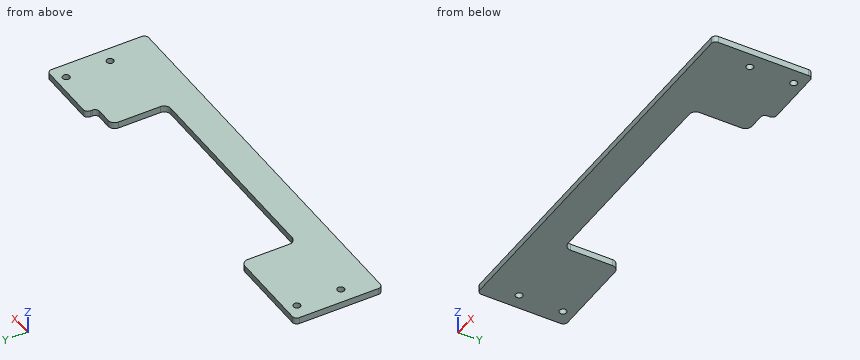
```python
from build123d import *

# Parameters (mm, degrees)
EXTRUDE_1_DEPTH     = 3
FILLET_1_R          = 2
SKETCH_2_R          = 1.6
CUT_EXTRUDE_1_DEPTH = 14
SKETCH_3_W          = 100
SKETCH_3_H          = 25
CUT_EXTRUDE_2_DEPTH = 14
FILLET_2_R          = 3


with BuildPart() as part:
    # 草图1 → 凸台-拉伸1 (new body)
    with BuildSketch(Plane.XY):
        Polygon((0, 0), (183.3, 0), (183.3, 40), (183.3, 45), (153.3, 45), (153.3, 40), (0, 40), align=None)
    extrude(amount=EXTRUDE_1_DEPTH)

    # 圆角1
    fillet_1_edges = [part.edges().sort_by_distance(p)[0] for p in [
        (0, 40, 1.5),
        (153.3, 40, 1.5),
        (153.3, 45, 1.5),
        (183.3, 45, 1.5),
        (183.3, 0, 1.5),
        (0, 0, 1.5),
    ]]
    fillet(fillet_1_edges, radius=FILLET_1_R)

    # 草图2 → 切除-拉伸1 (cut)
    with BuildSketch(Plane(origin=(0, 0, 0), x_dir=(-1, 0, 0), z_dir=(0, 0, -1))):
        with Locations((-176.3, 40.44)):
            Circle(SKETCH_2_R)
        with Locations((-176.3, 20.44)):
            Circle(SKETCH_2_R)
        with Locations((-7, 35)):
            Circle(SKETCH_2_R)
        with Locations((-7, 15)):
            Circle(SKETCH_2_R)
    extrude(amount=-CUT_EXTRUDE_1_DEPTH, mode=Mode.SUBTRACT)

    # 草图3 → 切除-拉伸2 (cut)
    with BuildSketch(Plane(origin=(0, 0, 0), x_dir=(-1, 0, 0), z_dir=(0, 0, -1))):
        with Locations((-91.65, 27.5)):
            Rectangle(SKETCH_3_W, SKETCH_3_H)
    extrude(amount=-CUT_EXTRUDE_2_DEPTH, mode=Mode.SUBTRACT)

    # 圆角2
    fillet_2_edges = [part.edges().sort_by_distance(p)[0] for p in [
        (141.65, 15, 1.5),
        (141.65, 40, 1.5),
        (41.65, 40, 1.5),
        (41.65, 15, 1.5),
    ]]
    fillet(fillet_2_edges, radius=FILLET_2_R)


solid = part.part
```
Design review of the part built by this model. Coordinates are the model's own, in mm. Coordinates: 2 decimals unless noted, no trailing zeros. Order: outer loops, then holes, each group sorted by start corner. A loop starts at its lowest first (then second) coordinate and runs counter-clockwise, first axis right, second up. Notation, with made-up numbers: M 70,-32.5 L 126,-32.5 A13 ccw 126,-26.5 Z; hole C 26.5,43.5 d3. An arc over 180 degrees is marked long. Answer as a JSON object with one key per item and string values. Group by question number.
1) Add section B-B, the plane y = 31. Write out the cut boundary in (x, z).
2) For pin 1 (1 mm diameter, centred on x = 117, z = 2.5, fed in from +Y); pin 2 (0.9 mm diameter, centred on x = 149, z = 1.5, fed in from +Y), all flat-tipped, find the tip position at first contact; note any pin that passes through.
3) Wall thickness on L1, parallel to Y at x = 176.3, z = 1.4; L2, parallel to X at y = 34.5, z = 1.7; L3, parallel to X at y = 34, z = 2.15: over which ranges is each line inside the solid? List them lowest first.
4) Add section A-A, the plane x = 7. Write out the cut boundary in (y, z).
5) Add section C-C, the plane z = 1.85. Write out the cut boundary in (x, y).
6) Add section D-D, the plane x = 176.3. Write out the cut boundary in (y, z), then the cut area to 3 significant figures.
Computed values:
{
 "1": {"outline": "M 0,0 L 41.65,0 L 41.65,3 L 0,3 Z; M 141.65,0 L 183.3,0 L 183.3,3 L 141.65,3 Z"},
 "2": {"pin 1": "stops at y = 15", "pin 2": "stops at y = 40"},
 "3": {"L1": "y = 0 to 18.84, 22.04 to 38.84, 42.04 to 45", "L2": "x = 0 to 5.48, 8.52 to 41.65, 141.65 to 183.3", "L3": "x = 0 to 5.75, 8.25 to 41.65, 141.65 to 183.3"},
 "4": {"outline": "M 0,0 L 13.4,0 L 13.4,3 L 0,3 Z; M 16.6,0 L 33.4,0 L 33.4,3 L 16.6,3 Z; M 36.6,0 L 40,0 L 40,3 L 36.6,3 Z"},
 "5": {"outline": "M 0,2 A2 ccw 2,0 L 181.3,0 A2 ccw 183.3,2 L 183.3,43 A2 ccw 181.3,45 L 155.3,45 A2 ccw 153.3,43 L 153.3,42 A2 cw 151.3,40 L 144.65,40 A3 ccw 141.65,37 L 141.65,18 A3 cw 138.65,15 L 44.65,15 A3 cw 41.65,18 L 41.65,37 A3 ccw 38.65,40 L 2,40 A2 ccw 0,38 Z; hole C 7,15 d3.2; hole C 7,35 d3.2; hole C 176.3,20.44 d3.2; hole C 176.3,40.44 d3.2"},
 "6": {"outline": "M 0,0 L 18.84,0 L 18.84,3 L 0,3 Z; M 22.04,0 L 38.84,0 L 38.84,3 L 22.04,3 Z; M 42.04,0 L 45,0 L 45,3 L 42.04,3 Z", "area": "116 mm^2"}
}
